Autodesk Inventor part; units mm, degrees
ref_plane "Start plane" through (0, 0, 0) normal (0, 0, 1) x (1, 0, 0)
ref_plane "End plane" through (0, 0, 651) normal (0, 0, 1) x (1, 0, 0)
ref_plane "Work Plane4" through (0, -20, 0) normal (0, 0.7071, -0.7071) x (1, 0, 0)
ref_plane "Start plane" through (0, 0, 0) normal (0, 0, 1) x (1, 0, 0)
ref_plane "End plane" through (0, 0, 651) normal (0, 0, 1) x (1, 0, 0)
sketch "Sketch" plane through (0, 0, 0) normal (0, 0, 1) x (1, 0, 0)
  line L0 (-20, -13.4) -> (-20, 13.4)
  line L1 (-13.4, 20) -> (13.4, 20)
  line L2 (20, 13.4) -> (20, -13.4)
  line L3 (13.4, -20) -> (-13.4, -20)
  arc A0 (-20, -13.4) -> (-13.4, -20) centre (-13.4, -13.4) ccw
  arc A1 (-13.4, 20) -> (-20, 13.4) centre (-13.4, 13.4) ccw
  arc A2 (20, 13.4) -> (13.4, 20) centre (13.4, 13.4) ccw
  arc A3 (13.4, -20) -> (20, -13.4) centre (13.4, -13.4) ccw
  arc A4 (-13.4, 17) -> (-17, 13.4) centre (-13.4, 13.4) ccw
  line L4 (-13.4, 17) -> (13.4, 17)
  arc A5 (17, 13.4) -> (13.4, 17) centre (13.4, 13.4) ccw
  line L5 (17, 13.4) -> (17, -13.4)
  arc A6 (13.4, -17) -> (17, -13.4) centre (13.4, -13.4) ccw
  line L6 (13.4, -17) -> (-13.4, -17)
  arc A7 (-17, -13.4) -> (-13.4, -17) centre (-13.4, -13.4) ccw
  line L7 (-17, -13.4) -> (-17, 13.4)
  line L8 (0, 22.0873) -> (0, -22.0873) construction
  line L9 (-22.0873, 0) -> (22.0873, 0) construction
  dimension "d7" = 6.6
  dimension "d10" = 40
  dimension "d11" = 40
  dimension "d12" = 3
  dimension "d15" = 20
  dimension "d16" = 20
extrude "Body" add sketch "Sketch" along normal up to surface (651 mm away) from surface at 0
sketch "Sketch3" plane through (0, 0, 0) normal (0, 0, 1) x (1, 0, 0)
  line L0 (0, 0) -> (10, 0)
ref_plane "Work Plane3" through (0, 0, 0) normal (0, -1, 0) x (1, 0, 0)
sketch "Sketch4" plane through (0, 0, 0) normal (0, -1, 0) x (1, 0, 0)
  line L0 (-2, 0) -> (12, 0)
  line L1 (-2, 651) -> (12, 651)
  dimension "d18" = 651
ref_plane "Work Plane4" through (0, -20, 0) normal (0, 0.7071, -0.7071) x (1, 0, 0)
split "Split1" plane through (0, -20, 0) removes the side toward (0, 0.7071, -0.7071)
ref_plane "Work Plane5" through (0, -20, 651) normal (0, 0.7071, 0.7071) x (1, 0, 0)
split "Split2" plane through (0, -20, 651) removes the side toward (0, 0.7071, 0.7071)
equation "\"d7\" = G_IR"
equation "\"d10\" = G_H"
equation "\"d11\" = G_W"
equation "\"d12\" = G_T"
equation "\"d15\" = 0.5 * d10"
equation "\"d16\" = 0.5 * d11"
equation "\"d3\" = G_L"
equation "\"G_W\" = 40"
equation "\"G_H\" = 40"
equation "\"G_T\" = 3"
equation "\"G_IR\" = 6.6"
equation "\"G_L\" = d18"
equation "\"G_OFFSET_START\" = 0"
equation "\"G_OFFSET_END\" = 0"
equation "\"d14\" = G_OFFSET_END + B_L"
equation "\"B_L\" = 651"
properties part number "DIN EN 10305-5 - 40 x 40 x 3  - 651" material "Steel, Mild"
Input: part model. Units: mm. Frame: model coordinates. A direction names the side the tool comes from. Round coordinates to 2 decimals unless told otherwise and drop trailing zeros. Loops run counter-clockwise (first coordinate to the right, second up) from the corner with the lowest first, then second, coordinate; pieces in that order, holes last. Notation, with made-up numbers: M 20,26.5 L 70,26.5 A17 ccw 70,37.5 Z; hole C 61,76.5 d7. An arc over 180 degrees is marked long. Answer as CSV lines item,"result". Start each with the question number.
(1) Section B-B, the plane y = -8. Output: boundary loops of the cut face in (x, z), plus the area to 3 significant figures.
(2) Draft query along Y for faces 3 (the flat face through (20, 0, 321)), 4 (the flat face through (0, 17, 321)), 5 (the flat face through (17.5, -0.3, 631.3)). Return one class per face: released by +Y, released by -Y, zero draft, split by the parting line, or undercut.
(3) Section C-C, the plane z = 602.5. Output: boundary loops of the cut face in (x, y).
(4) Section A-A, the plane x = 5.5. Output: boundary loops of the cut face in (y, z).
(5) First-contact query: pin 1 (4 mm diameter, centred on x = 13.5, y = -14, fed in from -Z). Flat tip, straight axial feed; report the tip coordinate or a pass-through.
(6) Line query: line 1 (X direction, y = -5.5, z = 403.5); line 2 (X direction, y = 14, z = 563.5). Output: solid intervals per line, ascending. Write a range as [from, to].
(7) Reachability of faces 1 (the flat face through (-17, 0, 321)), 2 (the flat face through (17.5, 0.3, 20.3)) from +Z, -Z, +X, -X, +Y, -Y: full face, straight path, thin tool, end or side. Return the list, or none.
Values found:
1,outline,"M -20,12 L -17,12 L -17,639 L -20,639 Z; M 17,12 L 20,12 L 20,639 L 17,639 Z"
1,area,"3,760 mm²"
2,face 3,"zero draft"
2,face 4,"undercut"
2,face 5,"released by +Y"
3,outline,"M -20,-13.4 A6.6 ccw -13.4,-20 L 13.4,-20 A6.6 ccw 20,-13.4 L 20,13.4 A6.6 ccw 13.4,20 L -13.4,20 A6.6 ccw -20,13.4 Z; hole M -17,-13.4 A3.6 ccw -13.4,-17 L 13.4,-17 A3.6 ccw 17,-13.4 L 17,13.4 A3.6 ccw 13.4,17 L -13.4,17 A3.6 ccw -17,13.4 Z"
4,outline,"M -20,0 L -17,3 L -17,648 L -20,651 Z; M 17,37 L 20,40 L 20,611 L 17,614 Z"
5,pin 1,"passes through"
6,line 1,"x = [-20, -17], [17, 20]"
6,line 2,"x = [-19.97, -16.95], [16.95, 19.97]"
7,face 1,"+Z, -Z"
7,face 2,"-Z, +X, -X, +Y"
